Work out the finished part from the listing and answer in its coordinate system (mm). Coordinates: 2 decimals unless noted, no trailing zeros. Order: outer loops, then holes, each group sorted by start corner. A loop starts at its lowest first (then second) coordinate and runs counter-clockwise, first axis right, second up.
```python
from build123d import *

# Parameters (mm, degrees)
F1_DEPTH = 3


with BuildPart() as f1:
    # F0 (on Front) → F1 (new body)
    with BuildSketch(Plane.XZ):
        with BuildLine():
            Line((-30.123222, 26.928305), (-30.123222, 41.928305))
            ThreePointArc((-30.123222, 41.928305), (-46.266543, 31.403405), (-46.028907, 12.133639))
            Line((-46.028907, 12.133639), (-45.373068, 11.055652))
            Line((-45.373068, 11.055652), (-32.285383, -10.456249))
            ThreePointArc((-32.285383, -10.456249), (-32.250589, -12.475808), (-33.99401, -13.495765))
            Line((-33.99401, -13.495765), (-42.436163, -13.495765))
            ThreePointArc((-42.436163, -13.495765), (-48.093017, -15.838911), (-50.436163, -21.495765))
            Line((-50.436163, -21.495765), (-50.436163, -24.992765))
            Line((-50.436163, -24.992765), (-23.436163, -24.992765))
            ThreePointArc((-23.436163, -24.992765), (-17.779309, -22.649619), (-15.436163, -16.992765))
            Line((-15.436163, -16.992765), (-15.436163, -13.992765))
            ThreePointArc((-15.436163, -13.992765), (-18.585945, -3.940307), (-16.190902, 6.318192))
            ThreePointArc((-16.190902, 6.318192), (-9.503928, 27.854266), (-27.123222, 41.928305))
            Line((-27.123222, 41.928305), (-27.123222, 26.928305))
            Line((-27.123222, 26.928305), (-30.123222, 26.928305))
        make_face()
        with BuildLine():
            Line((-45.373068, 11.055652), (-46.028907, 12.133639))
            ThreePointArc((-46.028907, 12.133639), (-45.709491, 11.589472), (-45.373068, 11.055652))
        make_face()
    extrude(amount=F1_DEPTH)


solid = f1.part
```
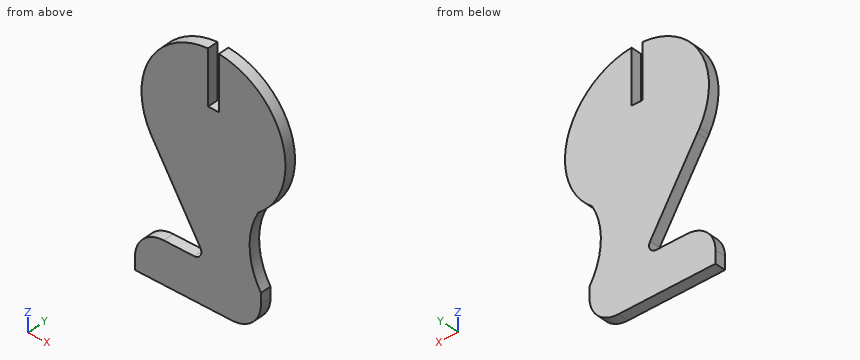
1. The part is cut by section B-B (x = -37.5). Determine the outline of the cut face in (y, z), plus the area to 3 significant figures.
2. The part is cut by section A-A (z = 34.5). Determine the outline of the cut face in (x, y), plus the area to 3 significant figures.
3. The part is cut by section C-C (y = -1.1). Determine the outline of the cut face in (x, z), plus the area to 3 significant figures.
4. The part is cut by section D-D (x = -28.5). Determine the outline of the cut face in (y, z), plus the area to 3 significant figures.
5. Consider probe 1 along Z at (x, y) = (-29.5, -2.25); probe 2 along X at (y, z) = (-1.25, 27.5); probe 3 along Z at (x, y) = (-38, -2.55). Determine where each line is inside the solid, lowest interval first.
6. Flat-ended cylindrical pins translate along their axes: pin 1 (0.9 mm diameter, centred on y = -1.5, z = 37, fed in from -X); pin 2 (1 mm diameter, centred on y = -1, z = 3.5, fed in from +X); pin 3 (1 mm diameter, centred on y = -1, z = 27.5, fed in from -X). Find the tip coordinate at first contact, or state that the pin passes through.
Worked out:
1. outline: (-3, -24.99) - (0, -24.99) - (0, -13.5) - (-3, -13.5) - close; (-3, -1.89) - (0, -1.89) - (0, 39.91) - (-3, 39.91) - close
1. area: 160 mm2
2. outline: (-44.22, -3) - (-30.12, -3) - (-30.12, 0) - (-44.22, 0) - close; (-27.12, -3) - (-13.02, -3) - (-13.02, 0) - (-27.12, 0) - close
2. area: 84.6 mm2
3. outline: (-50.44, -24.99) - (-23.44, -24.99) arc R8 ccw to (-15.44, -16.99) - (-15.44, -13.99) arc R20 cw to (-16.19, 6.32) arc R20 ccw to (-27.12, 41.93) - (-27.12, 26.93) - (-30.12, 26.93) - (-30.12, 41.93) arc R20 ccw to (-46.03, 12.13) arc R20 ccw to (-45.37, 11.06) - (-32.29, -10.46) arc R2 cw to (-33.99, -13.5) - (-42.44, -13.5) arc R8 ccw to (-50.44, -21.5) - close
3. area: 1,890 mm2
4. outline: (-3, -24.99) - (0, -24.99) - (0, 26.93) - (-3, 26.93) - close
4. area: 156 mm2
5. probe 1: z = -24.99 to 26.93
5. probe 2: x = -47.85 to -30.12, -27.12 to -9.4
5. probe 3: z = -24.99 to -13.5, -1.06 to 39.65
6. pin 1: stops at x = -42.33
6. pin 2: stops at x = -17.26
6. pin 3: stops at x = -47.98
